from build123d import *

# Parameters (mm, degrees)
F1_DEPTH = 10
F3_D     = 5
F3_DEPTH = 1
F3_TIP   = 1.5021515476
F5_D     = 5
F5_DEPTH = 1
F5_TIP   = 1.5021515476
F7_D     = 3
F9_D     = 3


with BuildPart() as f1:
    # F0 (on Front) → F1 (new body)
    with BuildSketch(Plane.XZ):
        Polygon((7.9454735894, 53.3583245364), (2.9454735894, 53.3583245364), (2.9454735894, 43.3583245364), (-27.4098654699, 13.0029854771), (-37.4098654699, 13.0029854771), (-37.4098654699, 8.0029854771), (-27.4098654699, 8.0029854771), (7.9454735894, 43.3583245364), align=None)
    extrude(amount=F1_DEPTH)

    # F3
    with Locations(Plane(origin=(2.9454735894, 0, 0), x_dir=(0, -1, 0), z_dir=(-1, 0, 0))):
        with Locations((5, 48.3583245364)):
            Hole(F3_D / 2, depth=F3_DEPTH)
            with Locations((0, 0, -(F3_DEPTH + F3_TIP / 2))):  # 118° drill point
                Cone(0, F3_D / 2, F3_TIP, mode=Mode.SUBTRACT)

    # F5
    with Locations(Plane.XY.offset(13.0029854771)):
        with Locations((-32.4098654699, -5)):
            Hole(F5_D / 2, depth=F5_DEPTH)
            with Locations((0, 0, -(F5_DEPTH + F5_TIP / 2))):  # 118° drill point
                Cone(0, F5_D / 2, F5_TIP, mode=Mode.SUBTRACT)

    # F7 (through all)
    with Locations(Plane.XY.offset(13.0029854771)):
        with Locations((-32.4098654699, -5)):
            Hole(F7_D / 2)

    # F9 (through all)
    with Locations(Plane(origin=(2.9454735894, 0, 0), x_dir=(0, -1, 0), z_dir=(-1, 0, 0))):
        with Locations((5, 48.3583245364)):
            Hole(F9_D / 2)


solid = f1.part
Can you work these out from the model? Positions are in its coordinate system, mm. A direction names the side the tool comes from. Round coordinates to 2 decimals unless told otherwise and drop trailing zeros. Write each loop counter-clockwise with the first axis right and the second up, starting at its lowest first coordinate (ties: lowest second). Pieces come first, ordered by that corner, then holes. Notation, with made-up numbers: (28.5, 40.5) -> (41.5, 40.5) arc R12 cw to (41.5, 57.5) -> close; hole circle Ø10 at (46, 49). An arc over 180 degrees is marked (long way). Use one line per item in the form item = value. Start each with the question number.
Q1. Imagine slicing it at B-B (x = -4.5). Please give me the cut outline in (y, z), then the cut area to 3 significant figures.
Q2. I'm going to push flat-ended pins straight in: P1, Ø6, axis at y = -5, z = 48.36, coming from the -X side; P2, Ø3, axis at y = -7.5, z = 41.5, coming from the +X side; P3, Ø5, axis at x = -34, y = -6, coming from the +Z side; P4, Ø8, axis at x = -9.5, z = 40.5, coming from the +Y side. Where does each tip first touch, or does it pass through?
Q3. Imagine slicing it at A-A (y = -5). Please give me the cut outline in (x, z).
Q4. If I drill on probe 1 along X at (y, z) = (-5, 9.5); probe 2 along X at (y, z) = (-3.5, 45); probe 3 along Y at (x, z) = (5.5, 47), over which ranges is the centre line in solid material (lowest first)? Write a range as [from, to].
Q5. Imagine slicing it at C-C (z = 28). Please give me the cut outline in (x, y), then the cut area to 3 significant figures.
Q6. We'd pull the mould along Y, two halves only. Please class faces 4 (the face through (-11, 0, 26)), 5 (the face through (3.452, -5.542, 45.918)), 6 (the face through (7.945, -4, 47)): +Y half, -Y half, draft (parallel to the pull), parting line (faces both ways), or undercut.
Q7. Which directions (+Z, -Z, +X, -X, +Y, -Y) give clear straight access to the entire face, cutting with the end or side of a thin tool? Please do faces 1 (the face through (-32.08, -2.52, 12.5)), 2 (the face through (-34, -4, 8.003)), 3 (the face through (-30, -3, 13.003)).
Worked out:
q1.outline = (-10, 30.91) -> (0, 30.91) -> (0, 35.91) -> (-10, 35.91) -> close
q1.area = 50.0 mm^2
q2.P1 = 2.95
q2.P2 = 7.59
q2.P3 = 13
q2.P4 = through
q3.outline = (-37.41, 8) -> (-33.91, 8) -> (-33.91, 11.4) -> (-34.91, 12) -> (-34.91, 13) -> (-37.41, 13) -> close; (-30.91, 8) -> (-27.41, 8) -> (7.95, 43.36) -> (7.95, 46.86) -> (4.55, 46.86) -> (3.95, 45.86) -> (2.95, 45.86) -> (2.95, 43.36) -> (-27.41, 13) -> (-29.91, 13) -> (-29.91, 12) -> (-30.91, 11.4) -> close; (2.95, 50.86) -> (3.95, 50.86) -> (4.55, 49.86) -> (7.95, 49.86) -> (7.95, 53.36) -> (2.95, 53.36) -> close
q4.probe_1 = [-37.41, -33.91], [-30.91, -25.91]
q4.probe_2 = [2.95, 7.95]
q4.probe_3 = [-10, -5.64], [-4.36, 0]
q5.outline = (-12.41, -10) -> (-7.41, -10) -> (-7.41, 0) -> (-12.41, 0) -> close
q5.area = 50.0 mm^2
q6.face_4 = +Y half
q6.face_5 = undercut
q6.face_6 = draft
q7.face_1 = +Z
q7.face_2 = -Z, +X, -X, +Y, -Y
q7.face_3 = +Z, -X, +Y, -Y
